CAD build for the part. Positions are in the model's coordinates, mm. Give positions to 0.01 mm unless a question says otherwise; leave off trailing zeros. Loops run counter-clockwise (first coordinate to the right, second up) from the corner with the lowest first, then second, coordinate; pieces in that order, holes last.
```python
from build123d import *

# Parameters (mm, degrees)
CANAL_C_3_X_5_1_DEPTH = 2100


with BuildPart() as part:
    # Sketch12 → Canal c 3 X 5(1) (new body)
    with BuildSketch(Plane(origin=(0, 0, 0), x_dir=(0, 0, -1), z_dir=(1, 0, 0))):
        with BuildLine():
            Line((0, -38.1), (0, 38.1))
            Line((0, 38.1), (38.0492, 38.1))
            Line((38.0492, 38.1), (38.0492, 35.942335136))
            ThreePointArc((38.0492, 35.942335136), (37.447280466, 34.300554363), (35.926803066, 33.436899509))
            Line((35.926803066, 33.436899509), (12.283671721, 29.496090157))
            ThreePointArc((12.283671721, 29.496090157), (8.178382741, 27.164222052), (6.5532, 22.731413966))
            Line((6.5532, 22.731413966), (6.5532, -22.731413966))
            ThreePointArc((6.5532, -22.731413966), (8.178382741, -27.164222052), (12.283671721, -29.496090157))
            Line((12.283671721, -29.496090157), (35.926803066, -33.436899509))
            ThreePointArc((35.926803066, -33.436899509), (37.447280466, -34.300554363), (38.0492, -35.942335136))
            Line((38.0492, -35.942335136), (38.0492, -38.1))
            Line((38.0492, -38.1), (0, -38.1))
        make_face()
    extrude(amount=CANAL_C_3_X_5_1_DEPTH)


solid = part.part
```
1. Saw through at C-C, the plane y = 6. List the corners of the cut face in (x, z).
Responses:
outline: (0, -6.55) - (2100, -6.55) - (2100, 0) - (0, 0) - close
2. Drop flat-ended pins along their axis: pin 1 (8 mm diameter, centred on x = 1385, y = 19, fed in from -Z); pin 2 (4 mm diameter, centred on x = 688, y = -23, fed in from -Z). Give the stop position or say it passes through.
Responses:
pin 1: stops at z = -6.56
pin 2: stops at z = -6.94
3. Saw through at A-A, the plane z = -28.5. List the corners of the cut face in (x, y), and give its area (3 significant figures).
Responses:
outline: (0, -38.1) - (2100, -38.1) - (2100, -32.2) - (0, -32.2) - close; (0, 32.2) - (2100, 32.2) - (2100, 38.1) - (0, 38.1) - close
area: 24,800 mm2
4. Probe line 1 along Y through (x, z) = (543, -11.5); line 2 along Y through (x, z) = (425, -12); line 3 along Z through (x, y) = (1702.5, 20). List the from-to ranges inside material, lowest first.
Responses:
line 1: y = -38.1 to -29.32, 29.32 to 38.1
line 2: y = -38.1 to -29.44, 29.44 to 38.1
line 3: z = -6.55 to 0
5. Saw through at B-B, the plane x = 201. List the corners of the cut face in (y, z), and give its area (3 significant figures).
Responses:
outline: (-38.1, -38.05) - (-35.94, -38.05) arc R2.54 ccw to (-33.44, -35.93) - (-29.5, -12.28) arc R6.86 cw to (-22.73, -6.55) - (22.73, -6.55) arc R6.86 cw to (29.5, -12.28) - (33.44, -35.93) arc R2.54 ccw to (35.94, -38.05) - (38.1, -38.05) - (38.1, 0) - (-38.1, 0) - close
area: 948 mm2
6. Pull direction Y, two halves, no side cores. Call faces 1 (the face through (1035, 0, -6.553)), 2 (the face through (0, 0, -6)), 3 (the face through (1035, 38.1, -19)): released by +Y, released by -Y, zero draft, split by the parting line, or undercut.
Responses:
face 1: undercut
face 2: zero draft
face 3: released by +Y
